Study the drawing (mm; zero at the part's minimum x, y, z) and answer. Coordinates: 2 decimals unless noted, no trailing zeros. Order: outer loops, then holes, each group sorted by start corner. A loop starts at its lowest first (then second) coordinate and runs counter-clockwise, first axis right, second up.
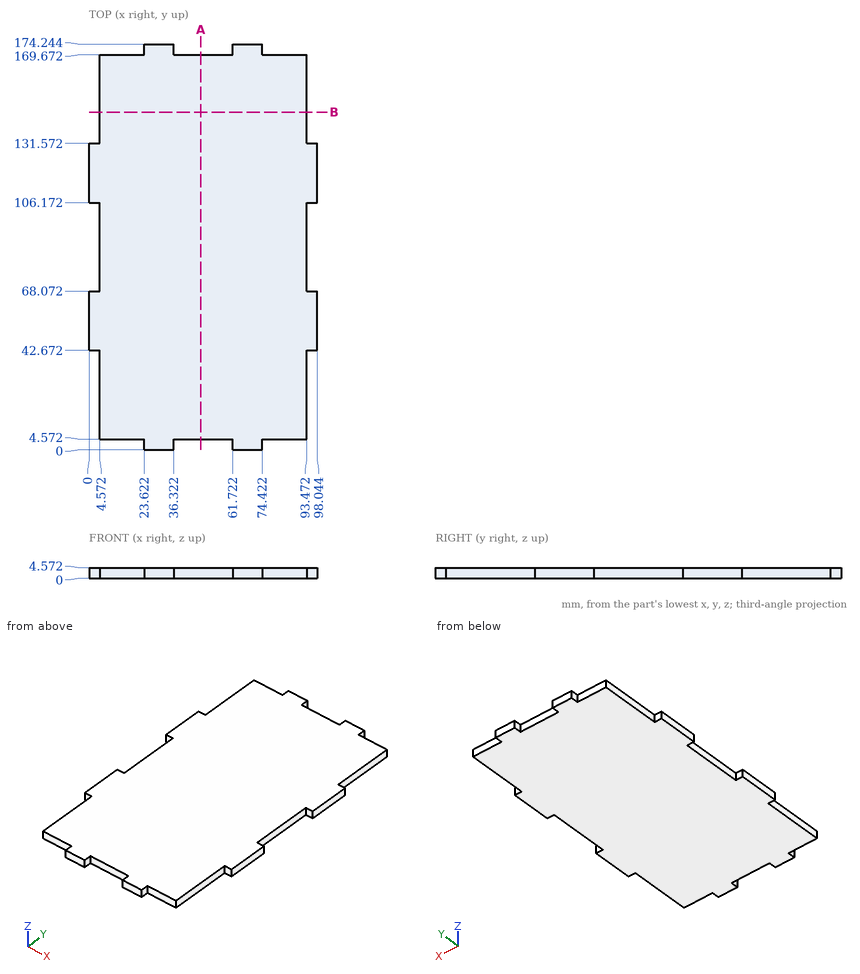
(1) Each of these flat-tipped pins is pushed along its axis until it touches: pin 1 Ø2.5 at (y, z) = (2, 3) entering from +X; pin 2 Ø2.5 at (y, z) = (151.5, 3) entering from -X; pin 3 Ø1.4 at (x, z) = (2, 3) entering from -Y. Where does it stop, or does it pass through?
(2) Consider line 1 (Y direction, x = 57.5, z = 3.1); line 2 (X direction, y = 99.5, z = 2.7). Determine where each line is inside the solid, lowest interval first.
(3) Find section B-B (y = 145). Write down the section's boundary in (x, z).
(4) Find section A-A (x = 48). Write down the section's boundary in (y, z).
Findings below:
1. pin 1: stops at x = 74.42
1. pin 2: stops at x = 4.57
1. pin 3: stops at y = 42.67
2. line 1: y = 4.57 to 169.67
2. line 2: x = 4.57 to 93.47
3. outline: (4.57, 0) - (93.47, 0) - (93.47, 4.57) - (4.57, 4.57) - close
4. outline: (4.57, 0) - (169.67, 0) - (169.67, 4.57) - (4.57, 4.57) - close
